from build123d import *

# Parameters (mm, degrees)
SKETCH1_R           = 9.5
BOSS_EXTRUDE1_DEPTH = 26
SKETCH5_W           = 14
SKETCH5_H           = 30
CUT_EXTRUDE2_DEPTH  = 57


with BuildPart() as part:
    # Sketch1 → Boss-Extrude1 (new body)
    with BuildSketch(Plane.XY):
        with BuildLine():
            Line((-15, 0), (-15, -34.753782032))
            Line((-15, -34.753782032), (35, -34.753782032))
            Line((35, -34.753782032), (35, -26.607408272))
            add(Edge.make_bspline(
                [(35, -26.607408272), (19.62178197, -24.621800081), (15, -15.829616288), (15, 0)],
                knots=[0, 0, 0, 0, 1, 1, 1, 1], degree=3))
            ThreePointArc((15, 0), (0, 15), (-15, 0))
        make_face()
        with Locations(Location((0, 0, 0), (0, 0, 180))):
            Circle(SKETCH1_R, mode=Mode.SUBTRACT)
    extrude(amount=BOSS_EXTRUDE1_DEPTH)

    # Sketch5 → Cut-Extrude2 (cut)
    with BuildSketch(Plane(origin=(17.578199992, 13.213011814, 0), x_dir=(0, 0, -1), z_dir=(0.7993586418199494, 0.6008541934178091, -6.982962677686267e-15))):
        with Locations((-13, 0)):
            Rectangle(SKETCH5_W, SKETCH5_H)
    extrude(amount=-CUT_EXTRUDE2_DEPTH, mode=Mode.SUBTRACT)


solid = part.part
Could you check a few things on this model? Use its own coordinates, in mm. A direction names the side the tool comes from. Give positions to 0.01 mm unless a question says otherwise; leave off trailing zeros. Order: outer loops, then holes, each group sorted by start corner. A loop starts at its lowest first (then second) coordinate and runs counter-clockwise, first axis right, second up. Notation, with made-up numbers: (8.5, -24) - (18.5, -24) arc R18 cw to (18.5, 9) - close; hole circle Ø1 at (-0.75, 85.5). An arc over 180 degrees is marked (long way). Return JSON: item names as keys, results as strings. Group by question number.
Q1. Please list where these lines run through material, in increasing order: line 1 along Y through (x, z) = (0, 2.75); line 2 along Z through (x, y) = (13.5, -8.5); line 3 along Y through (x, z) = (-1, 3.25). Write a range as [from, to].
Q2. Thinking about a two-plate mould opening in Z: for faces 1 (the face through (0.411, -18.456, 13.098)), 2 (the face through (4, -15, 26)), 3 (the face through (0, 15, 3)), which applies, pulls with the +Z half, pulls with the -Z half, needs draft (parallel to the pull), parting line crosses it, or undercut?
Q3. Suppose I cut it at A-A, the plane y = 6. Please give me the cut outline in (x, z).
Q4. Suppose I cut it at B-B, the plane x = 0. Please give me the cut outline in (y, z), and give its area (3 significant figures).
Q5. Which directions (+Z, -Z, +X, -X, +Y, -Y) give clear straight access to the entire face, cutting with the end or side of a thin tool? Please do faces 4 (the face through (-2, -10, 6)), 5 (the face through (35, -31, 13)).
Q6. Will these pins go through, and if not, where does the flat tip stop? pin 1 Ø17 at (x, y) = (0, 0) entering from +Z; pin 2 Ø10 at (y, z) = (-15.5, 12.5) entering from +X; pin 3 Ø10 at (x, z) = (27, 6.5) entering from +Y; pin 4 Ø3 at (y, z) = (2, 5.5) entering from +X.
Resolved:
{
 "1": {"line 1": "y = [-34.75, -9.5], [9.5, 15]", "line 2": "z = [0, 6], [20, 26]", "line 3": "y = [-34.75, -9.45], [9.45, 14.97]"},
 "2": {"face 1": "undercut", "face 2": "pulls with the +Z half", "face 3": "needs draft"},
 "3": {"outline": "(-13.75, 0) - (-7.37, 0) - (-7.37, 6) - (-13.75, 6) - close; (-13.75, 20) - (-7.37, 20) - (-7.37, 26) - (-13.75, 26) - close; (7.37, 0) - (13.75, 0) - (13.75, 6) - (7.37, 6) - close; (7.37, 20) - (13.75, 20) - (13.75, 26) - (7.37, 26) - close"},
 "4": {"outline": "(-34.75, 0) - (-9.5, 0) - (-9.5, 6) - (-18.77, 6) - (-18.77, 20) - (-9.5, 20) - (-9.5, 26) - (-34.75, 26) - close; (9.5, 0) - (15, 0) - (15, 6) - (9.5, 6) - close; (9.5, 20) - (15, 20) - (15, 26) - (9.5, 26) - close", "area": "593 mm2"},
 "5": {"face 4": "-X, +Y", "face 5": "+Z, -Z, +X, +Y, -Y"},
 "6": {"pin 1": "passes through", "pin 2": "stops at x = 20.87", "pin 3": "stops at y = -21.56", "pin 4": "stops at x = 14.99"}
}
